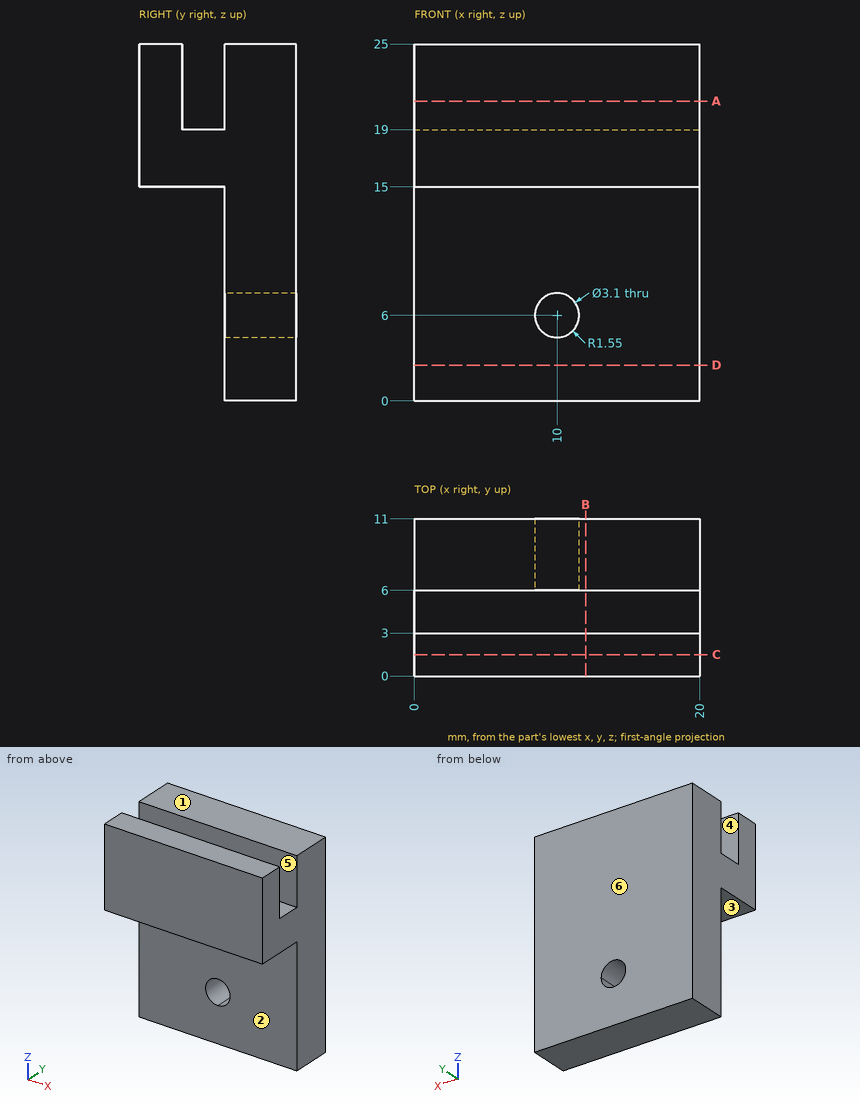
Geometry check sheet. Reference: drawing and pictorial views, mm from the part's lowest x, y, z. A direction names the side the tool comes from. Round coordinates to 2 decimals unless told otherwise and drop trailing zeros. Loops run counter-clockwise (first coordinate to the right, second up) from the corner with the lowest first, then second, coordinate; pieces in that order, holes last. Notation, with made-up numbers: M 0,31.5 L 46,31.5 A22 cw 46,62.5 Z; hole C 23.5,79.5 d8. An arc over 180 degrees is marked long. Return JSON: item names as keys, results as strings. Group by question number.
(1) Section check C-C, the plane y = 1.5. Enter the section's corners in (x, z).
(2) Section check D-D, the plane z = 2.5. Enter the section's corners in (x, y).
(3) Section check B-B, the plane x = 12. Enter the section's corners in (y, z).
(4) Go/stop test with flat-tipped pins: pin 1 (4 mm diameter, centred on x = 10, z = 6, fed in from -Y); pin 2 (2.5 mm diameter, centred on x = 12, y = 4.5, fed in from +Z). Record where each tip stops, or that it passes through.
(5) Scan lines: line 1 along X through (y, z) = (7.7, 6); line 2 along Z through (x, y) = (10, 9.95); line 3 along Y through (x, z) = (1.5, 23.75). Record each from-to range of solid material in increasing order. Write a range as [from, to].
(6) Set-up check for the marked faces 1 and 2: record each of +Z, -Z, +X, -X, +Y, -Y from which the full face is reachable in a straight line by a thin tool's end or side.
(7) Mould release check, pull along Y, two halves, no side actions. Record for the marked faces 3, 4, 5 and 6: pulls with the +Y half, pulls with the -Y half, needs draft (parallel to the pull), parting line crosses it, or undercut.
(8) Section check A-A, the plane z = 21. Enter the section's corners in (x, y), and give its area (3 significant figures).
Data:
{
 "1": {"outline": "M 0,15 L 20,15 L 20,25 L 0,25 Z"},
 "2": {"outline": "M 0,6 L 20,6 L 20,11 L 0,11 Z"},
 "3": {"outline": "M 0,15 L 6,15 L 6,0 L 11,0 L 11,25 L 6,25 L 6,19 L 3,19 L 3,25 L 0,25 Z"},
 "4": {"pin 1": "y = 6", "pin 2": "z = 19"},
 "5": {"line 1": "[0, 8.45], [11.55, 20]", "line 2": "[0, 4.45], [7.55, 25]", "line 3": "[0, 3], [6, 11]"},
 "6": {"face 1": "+Z, +X, -X, +Y, -Y", "face 2": "-Z, +X, -X, -Y"},
 "7": {"face 3": "needs draft", "face 4": "undercut", "face 5": "undercut", "face 6": "pulls with the +Y half"},
 "8": {"outline": "M 0,0 L 20,0 L 20,3 L 0,3 Z; M 0,6 L 20,6 L 20,11 L 0,11 Z", "area": "160 mm²"}
}
